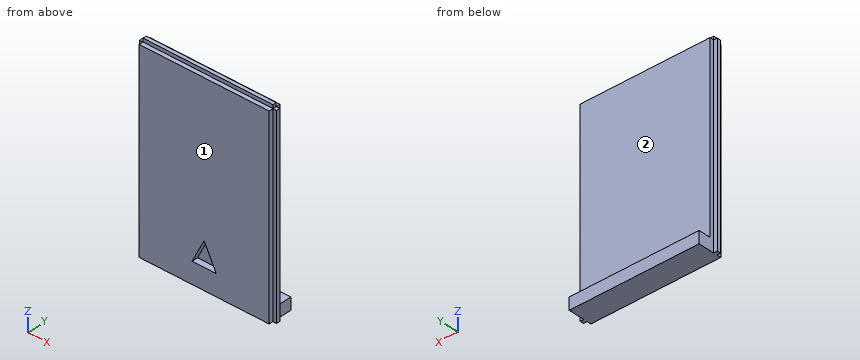
Autodesk Inventor part; units mm, degrees
ref_plane "YZ Plane" through (0, 0, 0) normal (1, 0, 0) x (0, 1, 0)
ref_plane "XZ Plane" through (0, 0, 0) normal (0, 1, 0) x (-1, 0, 0)
ref_plane "XY Plane" through (0, 0, 0) normal (0, 0, 1) x (1, 0, 0)
sketch "Esquisse1" plane through (0, 0, 0) normal (0, 1, 0) x (-1, 0, 0)
  line L0 (0, 0) -> (108, 0)
  line L1 (108, 0) -> (108, -160)
  line L2 (108, -160) -> (0, -160)
  line L3 (0, -160) -> (0, 0)
  dimension "d0" = 108
  dimension "d1" = 160
extrude "Extrusion1" add sketch "Esquisse1" along normal blind 10
sketch "Esquisse2" plane through (0, 10, 0) normal (0, 1, 0) x (1, 0, 0)
  line L0 (0, 160) -> (-108, 160)
  line L1 (-108, 160) -> (-108, 0)
  line L2 (0, 160) -> (-108, 160)
  line L3 (-108, 160) -> (-108, 150)
  line L4 (-108, 150) -> (0, 150)
  line L5 (0, 150) -> (0, 160)
  point P0 (0, 0)
  dimension "d4" = 10
extrude "Extrusion2" add sketch "Esquisse2" along normal blind 10
sketch "Esquisse3" plane through (0, 0, 0) normal (0, -1, 0) x (1, 0, 0)
  line L0 (-44, -142.4556) -> (-64, -142.4556)
  line L1 (0, 0) -> (0, -160)
  line L2 (-108, -160) -> (-108, 0)
  line L3 (-54, -122.4556) -> (-64, -142.4556)
  line L4 (-54, -122.4556) -> (-44, -142.4556)
  dimension "d7" = 20
  dimension "d8" = 44
  dimension "d9" = 44
extrude "Extrusion3" cut sketch "Esquisse3" against normal blind 5
sketch "Esquisse4" plane through (-108, 0, -160) normal (-1, 0, 0) x (0, 0, 1)
  line L0 (0, 0) -> (0, 20)
  line L1 (0, 6.5) -> (160, 6.5)
  line L2 (160, 0) -> (0, 0)
  line L3 (160, 6.5) -> (160, 3.5)
  line L4 (160, 3.5) -> (0, 3.5)
  line L5 (17.5444, 5) -> (37.5444, 5)
  line L6 (0, 3.5) -> (0, 6.5)
  point P0 (0, 3.5)
  dimension "d13" = 3
  dimension "d14" = 3.5
extrude "Extrusion4" add sketch "Esquisse4" along normal blind 3
sketch "Esquisse5" plane through (0, 0, 0) normal (1, 0, 0) x (0, 0, -1)
  line L0 (0, 3.5) -> (160, 3.5)
  line L1 (0, 3.5) -> (160, 3.5)
  line L2 (160, 6.5) -> (0, 6.5)
  line L3 (160, 3.5) -> (160, 6.5)
  line L4 (160, 6.5) -> (160, 3.5)
  line L5 (0, 6.5) -> (160, 6.5)
  line L6 (0, 6.5) -> (0, 3.5)
  line L7 (0, 0) -> (0, 10)
extrude "Extrusion5" add sketch "Esquisse5" along normal blind 3
sketch "Esquisse6" plane through (-108, 0, 0) normal (0, 0, 1) x (1, 0, 0)
  line L0 (0, 6.5) -> (-3, 6.5)
  line L1 (108, 6.5) -> (108, 10)
  line L2 (0, 6.5) -> (108, 6.5)
  line L3 (0, 3.5) -> (-3, 3.5)
  line L4 (108, 3.5) -> (0, 3.5)
  line L5 (0, 6.5) -> (0, 10)
  line L6 (0, 6.5) -> (0, 3.5)
  line L7 (108, 6.5) -> (108, 3.5)
  point P0 (108, 0)
extrude "Extrusion6" add sketch "Esquisse6" along normal blind 3
properties part number "couvercle pilier"
Model file for the job. Use its own axes, mm. Face numbers are marked on the shaded views. A direction names the side the tool comes from. Coordinates: 2 decimals unless noted, no trailing zeros. Loops run counter-clockwise (first coordinate to the right, second up) from the corner with the lowest first, then second, coordinate; pieces in that order, holes last. Notation, with made-up numbers: (59, 15.25) -> (84, 15.25) arc R19 cw to (84, 24.25) -> close; hole circle Ø6 at (18, -25). An arc over 180 degrees is marked (long way). Answer as a JSON object with one key per item and string values.
Q1. Cut at A-A (x = -67). List the corners of the cut face in (y, z).
Report:
{"outline": "(0, -160) -> (20, -160) -> (20, -150) -> (10, -150) -> (10, 0) -> (6.5, 0) -> (6.5, 3) -> (3.5, 3) -> (3.5, 0) -> (0, 0) -> close"}
Q2. Cut at D-D (x = -47). List the corners of the cut face in (y, z), and give its area (3 significant figures).
Report:
{"outline": "(0, -160) -> (20, -160) -> (20, -150) -> (10, -150) -> (10, 0) -> (6.5, 0) -> (6.5, 3) -> (3.5, 3) -> (3.5, 0) -> (0, 0) -> (0, -136.46) -> (5, -136.46) -> (5, -142.46) -> (0, -142.46) -> close", "area": "1,680 mm2"}
Q3. Cut at C-C (y = 17.75). List the corners of the cut face in (x, z), and give its area (3 significant figures).
Report:
{"outline": "(-108, -160) -> (0, -160) -> (0, -150) -> (-108, -150) -> close", "area": "1,080 mm2"}
Q4. 3-axis set-ups, long thin cutter, end or side, ignore diameter. For the marked faces 1 and 2: which of +Z, -Z, +X, -X, +Y, -Y reach the whole face in a straight line?
Report:
{"face 1": "+Z, -Z, +X, -X, -Y", "face 2": "+Z, +X, -X, +Y"}
Q5. Flat gauge pins, fed straight in: P1, Ø5, axis at x = -52, y = 13, coming from the +Z side; P2, Ø2.5, axis at x = -54, z = 2, coming from the -Y side; P3, Ø1, axis at y = 9.5, z = -78.5, coming from the +X side. Where does each tip first touch, or does it go through?
Report:
{"P1": "stops at z = -150", "P2": "stops at y = 3.5", "P3": "stops at x = 0"}
Q6. Probe probe 1 along Z at (x, y) = (-101.5, 17.25); probe 2 along Y at (x, z) = (-87.5, -139); probe 3 along X at (y, z) = (1.75, -54). List the from-to ranges inside material, lowest first.
Report:
{"probe 1": "z = -160 to -150", "probe 2": "y = 0 to 10", "probe 3": "x = -108 to 0"}
Q7. Cut at B-B (z = -56). List the corners of the cut face in (x, y), and give its area (3 significant figures).
Report:
{"outline": "(-111, 3.5) -> (-108, 3.5) -> (-108, 0) -> (0, 0) -> (0, 3.5) -> (3, 3.5) -> (3, 6.5) -> (0, 6.5) -> (0, 10) -> (-108, 10) -> (-108, 6.5) -> (-111, 6.5) -> close", "area": "1,100 mm2"}
